```python
from build123d import *

# Parameters (mm, degrees)
F0_W      = 69.85
F0_H      = 31.75
F1_DEPTH  = 25.4
F2_W      = 44.45
F2_H      = 25.4
F3_DEPTH  = 25.4
F4_R      = 12.69999
F5_R      = 6.35
F7_DEPTH  = 25.4
F8_DEPTH  = 25.4
F10_DEPTH = 25.4
F11_R     = 6.35
F12_DEPTH = 25.4
F14_DEPTH = 25.4


# Not quite as in the source:
# - a fillet or chamfer is up to 0.001 mm smaller than in the source, because OpenCascade refuses the exact size
# - ends of sketch curves that miss each other by under 0.0002 mm in the source are joined


with BuildPart() as f1:
    # F0 (on Front) → F1 (new body)
    with BuildSketch(Plane.XZ):
        with Locations((34.925, 15.875)):
            Rectangle(F0_W, F0_H)
    extrude(amount=F1_DEPTH)

    # F2 (on face) → F3 (cut)
    with BuildSketch(Plane.XZ.offset(25.4)):
        with Locations((47.625, 19.05)):
            Rectangle(F2_W, F2_H)
    extrude(amount=-F3_DEPTH, mode=Mode.SUBTRACT)

    # F4 (radius 12.7 in the source; OpenCascade refuses exactly that, so slightly less here)
    f4_edges = [f1.edges().sort_by_distance(p)[0] for p in [
        (25.4, -12.7, 31.75),
        (0, -12.7, 31.75),
    ]]
    fillet(f4_edges, radius=F4_R)

    # F5 (on face) → F7 (cut)
    with BuildSketch(Plane.XY.offset(6.35)):
        with Locations((38.1, -12.7)):
            Circle(F5_R)
    extrude(amount=-F7_DEPTH, mode=Mode.SUBTRACT)

    # F6 (on face) → F8 (cut)
    with BuildSketch(Plane.XY.offset(6.35)):
        with BuildLine():
            ThreePointArc((57.15, -19.05), (61.6401280605, -17.1901280605), (63.5, -12.7))
            ThreePointArc((63.5, -12.7), (61.6401280605, -8.2098719395), (57.15, -6.35))
            Line((57.15, -6.35), (38.1, -6.35))
            ThreePointArc((38.1, -6.35), (42.5901280605, -8.2098719395), (44.45, -12.7))
            ThreePointArc((44.45, -12.7), (42.7293038012, -17.046498167), (38.4997491919, -19.0374048777))
            Line((38.4997491919, -19.0374048777), (57.15, -19.05))
        make_face()
    extrude(amount=-F8_DEPTH, mode=Mode.SUBTRACT)

    # F9 (on face) → F10 (cut)
    with BuildSketch(Plane.XY.offset(6.35)):
        with BuildLine():
            ThreePointArc((63.8472363353, 0), (69.4711968718, -12.5871403191), (64.3824189901, -25.4))
            Line((64.3824189901, -25.4), (69.85, -25.4))
            Line((69.85, -25.4), (69.85, 0))
            Line((69.85, 0), (63.8472363353, 0))
        make_face()
    extrude(amount=-F10_DEPTH, mode=Mode.SUBTRACT)

    # F11 (on face) → F12 (cut)
    with BuildSketch(Plane.XZ.offset(25.4)):
        with Locations((12.7, 19.05)):
            Circle(F11_R)
    extrude(amount=-F12_DEPTH, mode=Mode.SUBTRACT)

    # F13 (on face) → F14 (cut)
    with BuildSketch(Plane.XY.offset(6.35)):
        with BuildLine():
            ThreePointArc((59.0771511197, 0), (69.1111732298, -12.7), (59.0771511197, -25.4))
            Line((59.0771511197, -25.4), (64.3824189901, -25.4))
            ThreePointArc((64.3824189901, -25.4), (69.4711968718, -12.5871403191), (63.8472363353, 0))
            Line((63.8472363353, 0), (59.0771511197, 0))
        make_face()
    extrude(amount=-F14_DEPTH, mode=Mode.SUBTRACT)


solid = f1.part
```
Design review of the part built by this model. Coordinates are the model's own, in mm. A direction names the side the tool comes from. Give positions to 0.01 mm unless a question says otherwise; leave off trailing zeros. Loops run counter-clockwise (first coordinate to the right, second up) from the corner with the lowest first, then second, coordinate; pieces in that order, holes last. Notation, with made-up numbers: (44.5, 4) -> (66.5, 4) arc R35 ccw to (66.5, 36) -> close; hole circle Ø4 at (-24.5, 59.5). An arc over 180 degrees is marked (long way). One line per item, written item: value.
Q1. Machinability: for faces 1 (the cylindrical face through (8.02, -12.88, 23.34)), 2 (the flat face through (25.4, -13, 13)), 3 (the cylindrical face through (31.75, -12.76, 3.22)), which of the approach directions +Z, -Z, +X, -X, +Y, -Y give a long, thin tool a straight path to every point of the face, cutting with its end or side? Answer none if there is none.
Numbers:
face 1: +Y, -Y
face 2: +Z, +X, +Y, -Y
face 3: +Z, -Z
Q2. For L1, parallel to Z at x = 12.7, y = -17; L2, parallel to X at y = -12.5, z = 11.5; L3, parallel to Z at x = 7.5, y = -7.5, list the stretches that pass through material, from the lowest coordinate up.
Numbers:
L1: z = 0 to 12.7, 25.4 to 31.75
L2: x = 0 to 25.4
L3: z = 0 to 15.41, 22.69 to 30.64
Q3. We need section B-B on x = 8. Give the boundary of the cut face in (y, z).
Numbers:
outline: (-25.4, 0) -> (0, 0) -> (0, 14.78) -> (-25.4, 14.78) -> close; (-25.4, 23.32) -> (0, 23.32) -> (0, 30.85) -> (-25.4, 30.85) -> close
Q4. Draft analysis for pull direction X (two halves, no side actions). For faces 4 (the flat face through (48, -6.35, 3)), 5 (the flat face through (47, -21, 6.35)), 6 (the cylindrical face through (3.62, -12.88, 27.93)), state which applies: pulls with the +X half, pulls with the -X half, needs draft (parallel to the pull), parting line crosses it, or undercut.
Numbers:
face 4: undercut
face 5: needs draft
face 6: pulls with the -X half
Q5. We need section C-C on y = -14.25. Give the number of separate pieces and of enclosed holes in the cut face, and give its area (3 significant figures).
Numbers:
separate pieces: 2
enclosed holes: 1
area: 688 mm^2
Q6. We need section A-A on z = 17. Give the boundary of the cut face in (x, y), and give its area (3 significant figures).
Numbers:
outline: (0, -25.4) -> (6.69, -25.4) -> (6.69, 0) -> (0, 0) -> close; (18.71, -25.4) -> (25.4, -25.4) -> (25.4, 0) -> (18.71, 0) -> close
area: 340 mm^2
Q7. For pin 1 Ø6 at (y, z) = (-4.5, 9.5) entering from +X; pin 2 Ø12.5 at (x, y) = (48.5, -9.5) entering from +Z; pin 3 Ø1 at (x, y) = (28.5, -11.5) entering from +Z, all flat-tipped, find the tip position at first contact; note any pin that passes through.
Numbers:
pin 1: stops at x = 25.4
pin 2: stops at z = 6.35
pin 3: stops at z = 6.35
